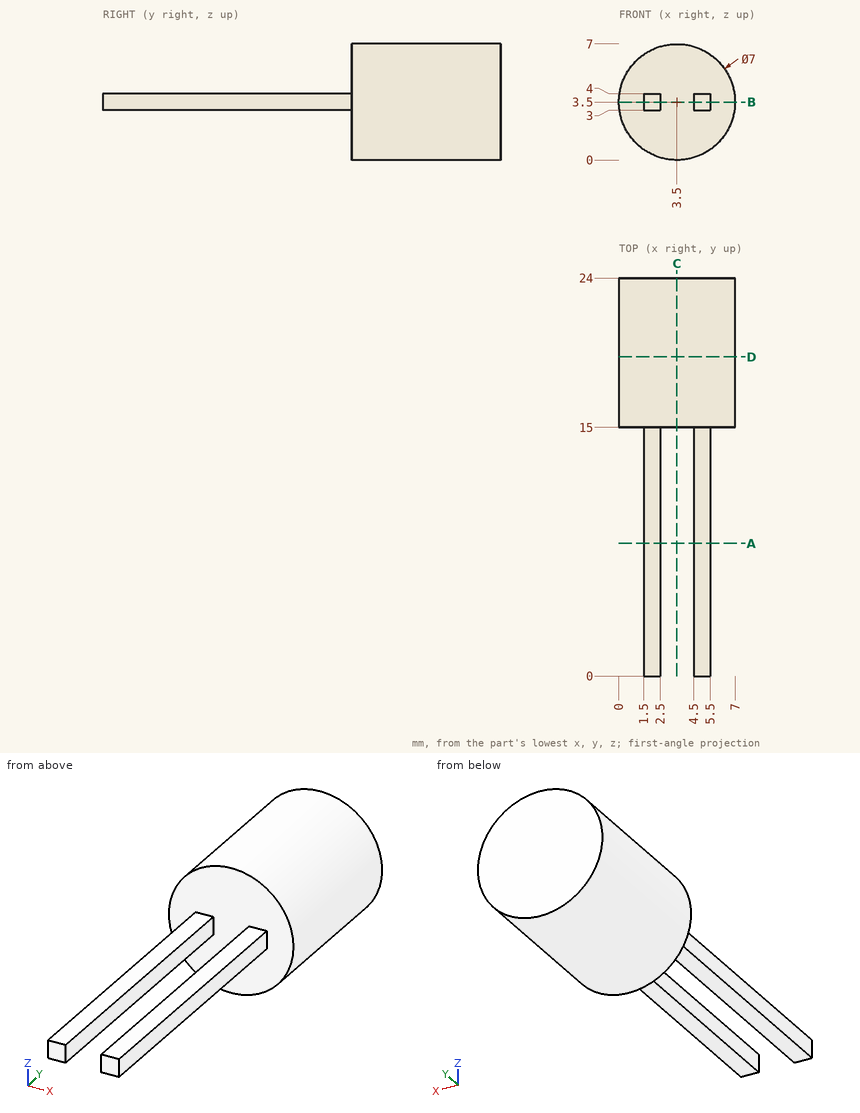
Geometry check sheet. Reference: drawing and pictorial views, mm from the part's lowest x, y, z. Round coordinates to 2 decimals unless told otherwise and drop trailing zeros. Loops run counter-clockwise (first coordinate to the right, second up) from the corner with the lowest first, then second, coordinate; pieces in that order, holes last.
1. Sectioned sample at B-B on z = 3.5. Record the boundary of the cut face in (x, y), and give its area (3 significant figures).
2. Sectioned sample at C-C on x = 3.5. Record the boundary of the cut face in (y, z).
3. Gauge pin test, flat ends, axial feed: pin 1 Ø0.5 at (y, z) = (11, 3.5) entering from +X; pin 2 Ø1.5 at (x, y) = (2.5, 12) entering from +Z; pin 3 Ø0.5 at (y, z) = (9, 3.5) entering from -X. Record the tip position at first contact, or that the pin passes through.
4. Sectioned sample at D-D on y = 19.25. Record the boundary of the cut face in (x, z), and give its area (3 significant figures).
5. Scan lines: probe 1 along Y at (x, z) = (6.5, 3.5); probe 2 along Z at (x, y) = (5, 9.25); probe 3 along Z at (x, y) = (1, 19.75). Record each from-to range of solid material in increasing order.
6. Sectioned sample at A-A on y = 8. Record the boundary of the cut face in (x, z), and give its area (3 significant figures).
Recorded:
1. outline: (0, 15) - (1.5, 15) - (1.5, 0) - (2.5, 0) - (2.5, 15) - (4.5, 15) - (4.5, 0) - (5.5, 0) - (5.5, 15) - (7, 15) - (7, 24) - (0, 24) - close
1. area: 93.0 mm2
2. outline: (15, 0) - (24, 0) - (24, 7) - (15, 7) - close
3. pin 1: stops at x = 5.5
3. pin 2: stops at z = 4
3. pin 3: stops at x = 1.5
4. outline: circle Ø7 at (3.5, 3.5)
4. area: 38.5 mm2
5. probe 1: y = 15 to 24
5. probe 2: z = 3 to 4
5. probe 3: z = 1.05 to 5.95
6. outline: (1.5, 3) - (2.5, 3) - (2.5, 4) - (1.5, 4) - close; (4.5, 3) - (5.5, 3) - (5.5, 4) - (4.5, 4) - close
6. area: 2.00 mm2
